The listing builds one solid part. Answer for the finished solid, in the listing's coordinates (mm). A direction names the side the tool comes from. Give positions to 0.01 mm unless a question says otherwise; leave off trailing zeros. Write each loop counter-clockwise with the first axis right and the second up, starting at its lowest first coordinate (ties: lowest second). Pieces come first, ordered by that corner, then holes.
```python
from build123d import *

# Parameters (mm, degrees)
F0_W     = 31.8008
F0_H     = 7.9502
F0_R     = 2.3876
F1_DEPTH = 3.175
F2_DEPTH = 4.7752
F3_T     = -1.6002


with BuildPart() as f1:
    # F0 (on Top) → F1 (new body)
    with BuildSketch(Plane.XY):
        with Locations((-4.8560211533, -2.5116165634)):
            Rectangle(F0_W, F0_H)
        with Locations((-16.7940211533, -2.1910497453)):
            Circle(F0_R, mode=Mode.SUBTRACT)
        with Locations((-8.8438211533, -2.1910497453)):
            Circle(F0_R, mode=Mode.SUBTRACT)
        with Locations((-0.8936211533, -2.1910497453)):
            Circle(F0_R, mode=Mode.SUBTRACT)
        with Locations((7.0565788467, -2.1910497453)):
            Circle(F0_R, mode=Mode.SUBTRACT)
    extrude(amount=F1_DEPTH)

    # F0 (on Top) → F2 (join)
    with BuildSketch(Plane.XY):
        with Locations((-16.7940211533, -2.1910497453)):
            Circle(F0_R)
        with Locations((-8.8438211533, -2.1910497453)):
            Circle(F0_R)
        with Locations((-0.8936211533, -2.1910497453)):
            Circle(F0_R)
        with Locations((7.0565788467, -2.1910497453)):
            Circle(F0_R)
    extrude(amount=F2_DEPTH)

    # F3
    f3_openings = [f1.faces().sort_by_distance(p)[0] for p in [
        (-4.856021, -2.511617, 0),
    ]]
    offset(amount=F3_T, openings=f3_openings, kind=Kind.INTERSECTION)


solid = f1.part
```
Item 1: A cutting plane is placed at D-D, the plane z = 3.5. Give the vertices of the cut face in (x, y).
Conclusion:
outline: circle Ø4.78 at (-16.79, -2.19); circle Ø4.78 at (-8.84, -2.19); circle Ø4.78 at (-0.89, -2.19); circle Ø4.78 at (7.06, -2.19)
Item 2: A cutting plane is placed at B-B, the plane x = -10.5. Give the vertices of the cut face in (y, z) (3 decimals), plus the area to 3 significant figures.
Conclusion:
outline: (-6.487, 0) - (-4.887, 0) - (-4.887, 1.575) - (-0.137, 1.575) - (-0.137, 0) - (1.463, 0) - (1.463, 3.175) - (-0.471, 3.175) - (-0.471, 4.775) - (-3.911, 4.775) - (-3.911, 3.175) - (-6.487, 3.175) - close
area: 23.3 mm2
Item 3: A cutting plane is placed at A-A, the plane z = 1.3. Give the vertices of the cut face in (x, y), plus the area to 3 significant figures.
Conclusion:
outline: (-20.76, -6.49) - (11.04, -6.49) - (11.04, 1.46) - (-20.76, 1.46) - close; hole (-19.16, -4.89) - (9.44, -4.89) - (9.44, -0.14) - (-19.16, -0.14) - close
area: 117 mm2
Item 4: Each of these flat-tipped pins is pushed along its axis until it touches: P1, Ø1.7, axis at x = -9, y = -2.5, coming from the -Z side; P2, Ø0.8, axis at x = -1, y = -2, coming from the -Z side (3 decimals); P3, Ø1, axis at x = -13.5, y = -3.5, coming from the +Z side (3 decimals). Where does it stop, or does it pass through?
Conclusion:
P1: stops at z = 1.57
P2: stops at z = 3.175
P3: stops at z = 3.175
Item 5: Consider probe 1 along Y at (x, z) = (3.5, 0.95); probe 2 along X at (y, z) = (-0.5, 0.5); probe 3 along Y at (x, z) = (-1, 2.1). Determine where each line is inside the solid, lowest interval first.
Conclusion:
probe 1: y = -6.49 to -4.89, -0.14 to 1.46
probe 2: x = -20.76 to -19.16, 9.44 to 11.04
probe 3: y = -6.49 to -2.97, -1.41 to 1.46
Item 6: Which of the six approach directions +Z, -Z, +X, -X, +Y, -Y give full straight-line access (tool end or side, diameter ignored) to faces 1 (the face through (-17, -2, 4.775)), 2 (the face through (6.27, -2.16, 2.36)), 3 (the face through (4.67, -2.09, 3.96))?
Conclusion:
face 1: +Z, +X, -X, +Y, -Y
face 2: -Z
face 3: +Z
Item 7: A cutting plane is placed at C-C, the plane y = -5.25. Give the vertices of the cut face in (x, z) (3 decimals), plus the area to 3 significant figures.
Conclusion:
outline: (-20.756, 0) - (11.044, 0) - (11.044, 3.175) - (-20.756, 3.175) - close
area: 101 mm2
Item 8: Determine the mould class of faces 4 (the face through (-5.1, -5.1, 0)), 5 (the face through (-5, -6.487, 2)), 6 (the face through (-5, -0.137, 1)) for opening direction Y: pulls with the +Y half, pulls with the -Y half, needs draft (parallel to the pull), parting line crosses it, or undercut.
Conclusion:
face 4: needs draft
face 5: pulls with the -Y half
face 6: undercut
